Read the model definition and answer for the solid it produces. Units are mm, in the model's axes. Coordinates: 2 decimals unless noted, no trailing zeros. Order: outer loops, then holes, each group sorted by start corner. A loop starts at its lowest first (then second) coordinate and runs counter-clockwise, first axis right, second up. Notation, with made-up numbers: M 5.5,-22.5 L 16.5,-22.5 A22 ccw 16.5,14.5 Z; hole C -33,66.5 d7. An arc over 180 degrees is marked long. Put each result on its own line as item: value.
from build123d import *

# Parameters (mm, degrees)
BOSS_EXTRUDE1_DEPTH = 1
FILLET2_R           = 3


with BuildPart() as part:
    # Sketch1 → Boss-Extrude1 (new body)
    with BuildSketch(Plane.XY):
        with BuildLine():
            Line((0, 0), (-15.859714544, -25.465063412))
            ThreePointArc((-15.859714544, -25.465063412), (-14.579001361, -30.975033806), (-9.069030967, -29.694320624))
            Line((-9.069030967, -29.694320624), (9.485017571, 0.096885346))
            Line((9.485017571, 0.096885346), (-9.673704642, 29.502871699))
            ThreePointArc((-9.673704642, 29.502871699), (-15.208686496, 30.670765479), (-16.376580276, 25.135783626))
            Line((-16.376580276, 25.135783626), (0, 0))
        make_face()
    extrude(amount=BOSS_EXTRUDE1_DEPTH)

    # Fillet2
    fillet2_edges = [part.edges().sort_by_distance(p)[0] for p in [
        (9.485017571, 0.096885346, 0.5),
        (0, 0, 0.5),
    ]]
    fillet(fillet2_edges, radius=FILLET2_R)


solid = part.part
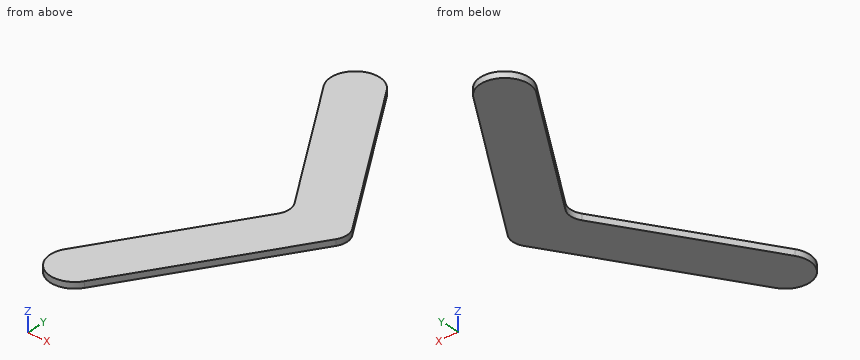
Q1. Find section D-D on y = -22.5. Write down the section's boundary in (x, z), plus the area to 3 significant figures.
Answers below:
outline: M -14.01,0 L -4.59,0 L -4.59,1 L -14.01,1 Z
area: 9.42 mm^2
Q2. Consider line 1 along Y through (x, z) = (-2, 0.8); line 2 along Y through (x, z) = (-5, 0.95); line 3 along Y through (x, z) = (3.75, 0.4). Determine where each line is inside the solid, lowest interval first.
Answers below:
line 1: y = -18.34 to -3.21, 3.07 to 17.72
line 2: y = -23.16 to -8.03, 7.67 to 22.33
line 3: y = -9.11 to 8.9
Q3. Find section B-B on z = 0.7. Write down the section's boundary in (x, y).
Answers below:
outline: M -16.38,25.14 L -1.04,1.6 A3 cw -1.01,-1.62 L -15.86,-25.47 A4 ccw -9.07,-29.69 L 8.47,-1.53 A3 ccw 8.44,1.7 L -9.67,29.5 A4 ccw Z
Q4. Find section C-C on x = -10.5. Write down the section's boundary in (y, z).
Answers below:
outline: M -31.06,0 L -16.86,0 L -16.86,1 L -31.06,1 Z; M 16.12,0 L 30.42,0 L 30.42,1 L 16.12,1 Z
Q5. Find section A-A on x = -5. Write down the section's boundary in (y, z).
Answers below:
outline: M -23.16,0 L -8.03,0 L -8.03,1 L -23.16,1 Z; M 7.67,0 L 22.33,0 L 22.33,1 L 7.67,1 Z
